The listing builds one solid part. Answer for the finished solid, in the listing's coordinates (mm). A direction names the side the tool comes from. Give positions to 0.01 mm unless a question says otherwise; leave off trailing zeros. Write each loop counter-clockwise with the first axis right and the second up, starting at its lowest first coordinate (ties: lowest second). Pieces come first, ordered by that corner, then holes. Notation, with made-up numbers: M 82,-33.5 L 123,-33.5 A20 cw 123,-15.5 Z; hole C -9,89 d1. An arc over 180 degrees is marked long. Return JSON: item names as keys, results as strings.
from build123d import *

# Parameters (mm, degrees)
SKETCH3_R          = 3
CUT_EXTRUDE1_DEPTH = 41.155946011


with BuildPart() as part:
    # Sketch2 → Revolve1 (revolve)
    with BuildSketch(Plane(origin=(0, 0, 0), x_dir=(1, 0, 0), z_dir=(0, 1, 0)), mode=Mode.PRIVATE) as revolve1_sk:
        Polygon((18.892201274, 8.5), (20.892201274, 8.5), (20.892201274, 15.5), (18.892201274, 17.5), (18.892201274, 27.5), (14.892201274, 27.5), (14.892201274, 17.5), (8.892201274, 17.5), (8.892201274, 14.5), (11.892201274, 14.5), (11.892201274, 13), (18.892201274, 13), align=None)
    revolve(revolve1_sk.sketch.rotate(Axis((0, 0, 0), (1, 0, 0)), 180), axis=Axis((0, 0, 0), (1, 0, 0)))

    # Sketch3 → Cut-Extrude1 (cut, through all)
    with BuildSketch(Plane(origin=(18.892201274, 0, 0), x_dir=(0, 0, -1), z_dir=(1, 0, 0))):
        with Locations((0, 22)):
            Circle(SKETCH3_R)
        with Locations((22, 0)):
            Circle(SKETCH3_R)
        with Locations((0, -22)):
            Circle(SKETCH3_R)
        with Locations((-22, 0)):
            Circle(SKETCH3_R)
    extrude(amount=-CUT_EXTRUDE1_DEPTH, mode=Mode.SUBTRACT)


solid = part.part
Item 1: Find the intervals of material crossed by line 1 (Y direction, x = 17.5, z = 0); line 2 (X direction, y = 11.5, z = 17); line 3 (X direction, y = -3.5, z = -8), in increasing order.
Geometry results:
{"line 1": "y = -27.5 to -25, -19 to -13, 13 to 19, 25 to 27.5", "line 2": "x = 14.89 to 18.89", "line 3": "x = 18.89 to 20.89"}
Item 2: A cutting plane is placed at A-A, the plane y = 0. Count the separate pieces of the cut face and the enclosed holes in it, plus the area to 3 significant figures.
Geometry results:
{"separate pieces": "4", "enclosed holes": "0", "area": "145 mm2"}
Item 3: Determine the mould class of faces 4 (the flat face through (8.892, -13, -7)), 5 (the cylindrical face through (11.85, 17.084, -3.794)), 6 (the cylindrical face through (16.92, -24.93, 0.65)) for opening direction Z: +Z half, -Z half, draft (parallel to the pull), parting line (faces both ways), or undercut.
Geometry results:
{"face 4": "draft", "face 5": "parting line", "face 6": "undercut"}
Item 4: A cutting plane is placed at B-B, the plane z = 22. Write down the section's boundary in (x, y), plus the area to 3 significant figures.
Geometry results:
{"outline": "M 14.89,-16.5 L 18.89,-16.5 L 18.89,-3 L 14.89,-3 Z; M 14.89,3 L 18.89,3 L 18.89,16.5 L 14.89,16.5 Z", "area": "108 mm2"}
Item 5: A cutting plane is placed at D-D, the plane x = 16. Write down the section's boundary in (y, z).
Geometry results:
{"outline": "C 0,0 d55; hole C -22,0 d6; hole C 0,0 d26; hole C 0,-22 d6; hole C 0,22 d6; hole C 22,0 d6"}
Item 6: Given pin 1 Ø16.5 at (y, z) = (0.5, -7) entering from +X; pin 2 Ø7 at (y, z) = (22, 0) entering from -X; pin 3 Ø4 at (x, z) = (19, 16) entering from +Y; pin 4 Ø4 at (x, z) = (10, 16) entering from -Y, each flat-ended and moving along its own axis, determine where each tip first touches the part or whether it passes through.
Geometry results:
{"pin 1": "stops at x = 20.89", "pin 2": "stops at x = 14.89", "pin 3": "stops at y = 23.67", "pin 4": "stops at y = -10.5"}
Item 7: Which of the six approach directions +Z, -Z, +X, -X, +Y, -Y give full straight-line access (tool end or side, diameter ignored) to faces 1 (the flat face through (14.892, 18, 0)), 2 (the cylindrical face through (17, 0, 25)), 3 (the flat face through (18.892, 0, -18))?
Geometry results:
{"face 1": "-X", "face 2": "+X, -X", "face 3": "+X"}
